The model under review builds one solid part; all positions refer to its coordinate system, in mm. Face numbers are marked on the shaded views. A direction names the side the tool comes from. Round coordinates to 2 decimals unless told otherwise and drop trailing zeros.
Item 1: Machinability: for the marked faces 1 and 2, which of the approach directions +Z, -Z, +X, -X, +Y, -Y give a long, thin tool a straight path to every point of the face, cutting with its end or side? Answer none if there is none.
Item 2: Clearance check with flat-ended pins moving along their axes: pin 1 Ø2 at (x, y) = (0, 0) entering from -Z; pin 2 Ø3 at (y, z) = (2, 10.5) entering from -X. State where each tip first meets the part, or that it passes through.
Item 3: To check wall thickness, follow L1, parallel to Y at x = 0, z = 11.25; L2, parallel to Y at x = -1, z = 6.25; L3, parallel to X at y = 1.5, z = 4. State the ranges of each line that lie inside material, in increasing order.
Item 4: Draft analysis for pull direction Y (two halves, no side actions). For the marked faces 3, 4, 5 and 6, state which applies: +Y half, -Y half, draft (parallel to the pull), parting line (faces both ways), or undercut.
Autodesk Inventor part; units mm, degrees
ref_plane "Work Plane1" through (-1.711, 0.0003, 0) normal (0, 1, 0) x (1, 0, 0)
ref_plane "Work Plane2" through (0.1135, 0.0003, 6.35) normal (0, 0, -1) x (-1, 0, 0)
ref_plane "YZ Plane" through (0, 0, 0) normal (1, 0, 0) x (0, 1, 0)
sketch "Sketch1" plane through (0, 0, 0) normal (0, 0, 1) x (1, 0, 0)
  line L0 (1.9552, -3.1747) -> (-1.711, -3.1747)
  line L1 (-1.711, -3.1747) -> (-3.5441, 0.0003)
  line L2 (-3.5441, 0.0003) -> (-1.711, 3.1753)
  line L3 (-1.711, 3.1753) -> (1.9552, 3.1753)
  line L4 (1.9552, 3.1753) -> (3.7883, 0.0003)
  line L5 (3.7883, 0.0003) -> (1.9552, -3.1747)
  point P0 (0.1221, 0.0003)
  dimension "d0" = 6.35
extrude "Extrusion1" add sketch "Sketch1" along normal blind 12.7
ref_plane "Work Plane1" through (-1.711, 0.0003, 0) normal (0, 1, 0) x (1, 0, 0)
sketch "Sketch3" plane through (-1.711, 0.0003, 0) normal (0, 1, 0) x (1, 0, 0)
  line L0 (-1.3251, 0) -> (4.9741, 0)
  line L1 (5.4821, -0.508) -> (5.4821, -12.192)
  line L2 (-1.8331, -12.192) -> (-1.8331, -0.508)
  line L3 (-1.8331, -0.508) -> (-1.3251, 0)
  line L4 (4.9741, 0) -> (5.4821, -0.508)
  line L5 (-1.8331, 0) -> (-1.8331, -12.7)
  line L6 (3.6662, 0) -> (5.4993, 0)
  line L7 (1.8245, 0) -> (1.8245, -12.7)
  line L8 (0, -12.7) -> (-1.8331, -12.7)
  line L9 (5.4993, -12.7) -> (3.6662, -12.7)
  line L10 (3.6662, -12.7) -> (0, -12.7)
  line L11 (-1.3251, -12.7) -> (-1.8331, -12.192)
  line L12 (4.9741, -12.7) -> (5.4821, -12.192)
  point P0 (-1.8331, 0)
  point P1 (5.4821, 0)
  point P2 (5.4821, -12.7)
  dimension "d5" = 0.508
  dimension "d6" = 0.508
  dimension "d7" = 0.508
  dimension "d8" = 0.508
  dimension "d16" = 0
  dimension "d46" = 0.508
  dimension "d47" = 0.508
  dimension "d48" = 0.508
  dimension "d49" = 0.508
revolve "Revolution1" cut sketch "Sketch3" angle 360 about axis through (0.1135, 0.0003, 0) along (0, 0, 1) keep common part contours L0 L4 L1 L12 L9 L10 L7
sketch "Sketch6" plane through (0.1135, 0.0003, 0) normal (0, 0, -1) x (-1, 0, 0)
  circle A0 centre (0, 0) radius 3.1496
hole "Hole3" at (0.1135, 0.0003, 0) direction (0, 0, 1) diameter 3.302 depth 6.35 tip angle 118
sketch "Sketch7" plane through (0, 0, 12.7) normal (0, 0, 1) x (1, 0, 0)
  point P0 (0, 0)
hole "Hole4" at (0, 0, 12.7) direction (0, 0, -1) diameter 3.302 depth 6.35 tip angle 118
ref_plane "Work Plane2" through (0.1135, 0.0003, 6.35) normal (0, 0, -1) x (-1, 0, 0)
properties part number "0.5 inch Standoff" material "Steel"
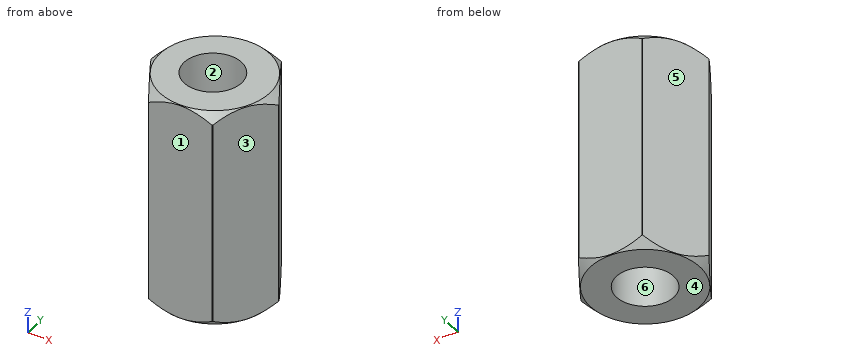
Numbers:
1. face 1: +Z, -Z, +X, -X, -Y
1. face 2: +Z
2. pin 1: passes through
2. pin 2: stops at x = -3.26
3. L1: y = -3.17 to -1.65, 1.65 to 3.18
3. L2: y = -3.17 to -1.22, 1.22 to 3.18
3. L3: x = -2.68 to -0.58, 0.8 to 2.92
4. face 3: -Y half
4. face 4: draft
4. face 5: +Y half
4. face 6: undercut
